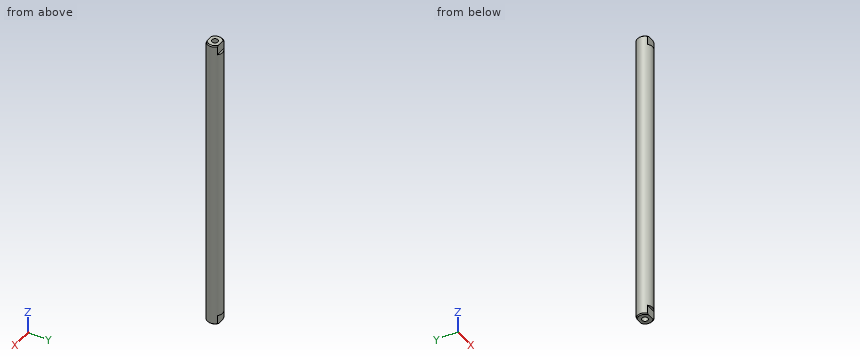
```python
from build123d import *

# Parameters (mm, degrees)
SKETCH1_R           = 3.175
BOSS_EXTRUDE1_DEPTH = 63.119
CHAMFER1_SIZE       = 0.381
CUT_EXTRUDE1_DEPTH  = 3.96875


with BuildPart() as part:
    # Sketch1 → Boss-Extrude1 (new body, symmetric)
    with BuildSketch(Plane.XY):
        Circle(SKETCH1_R)
    extrude(amount=BOSS_EXTRUDE1_DEPTH, both=True)

    # Sketch4 → M3x0.5 Tapped Hole1 (revolve, cut)
    with BuildSketch(Plane(origin=(0, 0, 63.119), x_dir=(0, -1, 0), z_dir=(1, 0, 0))):
        Polygon((0, 0), (0, 8.244075774), (1.25, 7.493), (1.25, 0), align=None)
    m3x0_5_tapped_hole1 = revolve(axis=Axis((0, 0, 69.469), (0, 0, -1)), mode=Mode.SUBTRACT)

    # Chamfer1
    chamfer1_edges = [part.edges().sort_by_distance(p)[0] for p in [
        (-3.175, 0, -63.119),
        (-3.175, 0, 63.119),
    ]]
    chamfer(chamfer1_edges, length=CHAMFER1_SIZE)

    # Mirror1: M3x0.5 Tapped Hole1 across plane
    add(m3x0_5_tapped_hole1.mirror(Plane.XY), mode=Mode.SUBTRACT)

    # Sketch5 → Cut-Extrude1 (cut)
    with BuildSketch(Plane.XY.offset(63.119)):
        with BuildLine():
            Line((-2.100065103, 2.38125), (2.100065103, 2.38125))
            ThreePointArc((2.100065103, 2.38125), (0, 3.175), (-2.100065103, 2.38125))
        make_face()
        with BuildLine():
            Line((-2.100065103, -2.38125), (2.100065103, -2.38125))
            ThreePointArc((2.100065103, -2.38125), (0, -3.175), (-2.100065103, -2.38125))
        make_face()
    cut_extrude1 = extrude(amount=-CUT_EXTRUDE1_DEPTH, mode=Mode.SUBTRACT)

    # Mirror2: Cut-Extrude1 across plane
    add(cut_extrude1.mirror(Plane.XY), mode=Mode.SUBTRACT)


solid = part.part
```
Source: CAD feature listing. Evaluate the final solid. Frame: model axes, mm. Coordinates: 2 decimals unless noted, no trailing zeros. Order: outer loops, then holes, each group sorted by start corner. A loop starts at its lowest first (then second) coordinate and runs counter-clockwise, first axis right, second up. Notation, with made-up numbers: (21.5, -9) - (76.5, -9) arc R17 cw to (76.5, 23) - close; hole circle Ø1 at (54, 22.5). An arc over 180 degrees is marked (long way). One line per item, written item: value.
1) Cut plane A-A on z = 48. Output: boundary loops of the cut face in (x, y) (3 decimals), plus the area to 3 significant figures.
Computed values:
outline: circle Ø6.35 at (0, 0)
area: 31.7 mm^2
2) Ray query, line 1 (X direction, y = 0, z = -58) (3 decimals); line 2 (Z direction, x = 1.5, y = 2.5); line 3 (X direction, y = -1.5, z = -24.5). Return the intervals inside material, ascending. Write a range as [from, to].
Computed values:
line 1: x = [-3.175, -1.25], [1.25, 3.175]
line 2: z = [-59.15, 59.15]
line 3: x = [-2.8, 2.8]
3) Contact query for flat-ended pins moving along their axis: pin 1 (3 mm diameter, centred on x = 0, z = 61.5, fed in from +Y); pin 2 (0.6 mm diameter, centred on x = 0, y = 3, fed in from -Z); pin 3 (1.2 mm diameter, centred on x = -1, z = 62, fed in from -Y). Output: stop coordinate, or through.
Computed values:
pin 1: stops at y = 2.38
pin 2: stops at z = -59.15
pin 3: stops at y = -2.38
